Source: CAD feature listing. Evaluate the final solid. Frame: model axes, mm. Give positions to 0.01 mm unless a question says otherwise; leave off trailing zeros. Order: outer loops, then holes, each group sorted by start corner. A loop starts at its lowest first (then second) coordinate and runs counter-clockwise, first axis right, second up.
1) Material intervals for line 1 (Z direction, x = 0, y = -2.8); line 2 (Z direction, x = -1.25, y = -1.65); line 3 (Y direction, x = -1.25, z = 36), sorted ascending.
2) Section A-A, the plane z = 167.5. Return loops of the section in (x, y), plus the area to 3 significant figures.
3) First-contact query: P1, Ø1.5, axis at y = -1.5, z = 185.5, coming from the +X side; P2, Ø2, axis at x = 0.5, z = 66.5, coming from the +Y side; P3, Ø1.5, axis at y = -2, z = 126, coming from the -X side; P4, Ø0.9, axis at y = -2.5, z = 64.5, coming from the +X side. Flat tips, straight axial feed; report the tip coordinate or a pass-through.
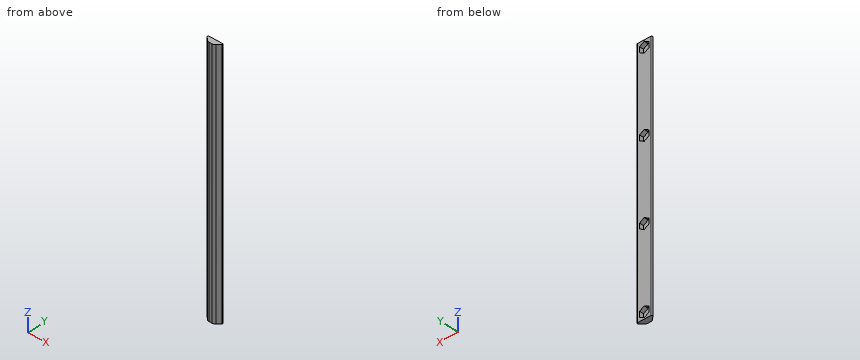
```python
from build123d import *

# Parameters (mm, degrees)
BOSS_EXTRUDE1_DEPTH = 190
CUT_EXTRUDE1_DEPTH  = 3.2


with BuildPart() as part:
    # Sketch1 → Boss-Extrude1 (new body)
    with BuildSketch(Plane(origin=(0, 0, 0), x_dir=(-1, 0, 0), z_dir=(0, 0, 1))):
        with BuildLine():
            Line((-1.134570377, 4.387902266), (1.134570572, 4.387902266))
            ThreePointArc((1.134570572, 4.387902266), (2.22521788, 4.17095913), (3.149824172, 3.553157318))
            Line((3.149824172, 3.553157318), (5.489602344, 1.213380832))
            ThreePointArc((5.489602344, 1.213380832), (5.624633323, 0.534535222), (5.049135806, 0.15))
            Line((5.049135806, 0.15), (-5.049135806, 0.15))
            ThreePointArc((-5.049135806, 0.15), (-5.624631872, 0.534534102), (-5.489601617, 1.213377992))
            Line((-5.489601617, 1.213377992), (-3.149825429, 3.553155866))
            ThreePointArc((-3.149825429, 3.553155866), (-2.225218633, 4.170958737), (-1.134570377, 4.387902266))
        make_face()
    extrude(amount=BOSS_EXTRUDE1_DEPTH)

    # Sketch2 → Cut-Extrude1 (cut)
    with BuildSketch(Plane(origin=(0, -0.15, 0), x_dir=(1, 0, 0), z_dir=(0, 1, 0))):
        Polygon((0, -0.929680602), (-3.525, -2.964840301), (-3.525, -7.035159699), (0, -9.070319398), (3.525, -7.035159699), (3.525, -2.964840301), align=None)
        Polygon((0, -60.929680602), (-3.525, -62.964840301), (-3.525, -67.035159699), (0, -69.070319398), (3.525, -67.035159699), (3.525, -62.964840301), align=None)
        Polygon((0, -120.929680602), (-3.525, -122.964840301), (-3.525, -127.035159699), (0, -129.070319398), (3.525, -127.035159699), (3.525, -122.964840301), align=None)
        Polygon((0, -180.929680602), (-3.525, -182.964840301), (-3.525, -187.035159699), (0, -189.070319398), (3.525, -187.035159699), (3.525, -182.964840301), align=None)
    extrude(amount=-CUT_EXTRUDE1_DEPTH, mode=Mode.SUBTRACT)


solid = part.part
```
From the geometry:
1. line 1: z = 0 to 0.93, 9.07 to 60.93, 69.07 to 120.93, 129.07 to 180.93, 189.07 to 190
1. line 2: z = 0 to 1.65, 8.35 to 61.65, 68.35 to 121.65, 128.35 to 181.65, 188.35 to 190
1. line 3: y = -4.39 to -0.15
2. outline: (-5.49, -1.21) - (-3.15, -3.55) arc R2.85 ccw to (-1.13, -4.39) - (1.13, -4.39) arc R2.85 ccw to (3.15, -3.55) - (5.49, -1.21) arc R0.62 ccw to (5.05, -0.15) - (-5.05, -0.15) arc R0.62 ccw to start
2. area: 36.3 mm2
3. P1: stops at x = 5.67
3. P2: stops at y = -3.35
3. P3: stops at x = -5.45
3. P4: stops at x = 4.65
